```python
from build123d import *

# Parameters (mm, degrees)
SKETCH1_W           = 25
SKETCH1_H           = 25
SKETCH1_R           = 6.5
BOSS_EXTRUDE1_DEPTH = 13
FILLET1_R           = 1.5


with BuildPart() as part:
    # Sketch1 → Boss-Extrude1 (new body)
    with BuildSketch(Plane.XY):
        Rectangle(SKETCH1_W, SKETCH1_H)
        with Locations(Location((0, 0, 0), (0, 0, 180))):
            Circle(SKETCH1_R, mode=Mode.SUBTRACT)
    extrude(amount=BOSS_EXTRUDE1_DEPTH)

    # Fillet1
    fillet1_edges = [part.edges().sort_by_distance(p)[0] for p in [
        (6.5, 0, 13),
    ]]
    fillet(fillet1_edges, radius=FILLET1_R)


solid = part.part
```
Verification items for the finished model (mm, model axes). Round coordinates to 2 decimals unless told otherwise and drop trailing zeros. Order: outer loops, then holes, each group sorted by start corner. A loop starts at its lowest first (then second) coordinate and runs counter-clockwise, first axis right, second up.
1) Cross-section at C-C, the plane z = 2. Record the cut outline in (x, y), plus the area to 3 significant figures.
Geometry says:
outline: (-12.5, -12.5) - (12.5, -12.5) - (12.5, 12.5) - (-12.5, 12.5) - close; hole circle Ø13 at (0, 0)
area: 492 mm2
2) Material ranges on line 1 (Y direction, x = 0, z = 4.75); line 2 (X direction, y = 0.5, z = 7.5); line 3 (X direction, y = 1, z = 12.5), recorded low to high.
Geometry says:
line 1: y = -12.5 to -6.5, 6.5 to 12.5
line 2: x = -12.5 to -6.48, 6.48 to 12.5
line 3: x = -12.5 to -6.81, 6.81 to 12.5
3) Cross-section at A-A, the plane y = 0. Record the cut outline in (x, z).
Geometry says:
outline: (-12.5, 0) - (-6.5, 0) - (-6.5, 11.5) arc R1.5 ccw to (-8, 13) - (-12.5, 13) - close; (6.5, 0) - (12.5, 0) - (12.5, 13) - (8, 13) arc R1.5 ccw to (6.5, 11.5) - close
4) Draft check along X on faces 1 (the flat face through (-12.5, 0, 6)), 2 (the flat face through (12.5, 0, 6)), 3 (the cylindrical face through (5.158, 3.955, 5.67)), 4 (the flat face through (-6, 6, 0)). Enter one of: +X half, -X half, draft (parallel to the pull), parting line (faces both ways), or undercut.
Geometry says:
face 1: -X half
face 2: +X half
face 3: undercut
face 4: draft
